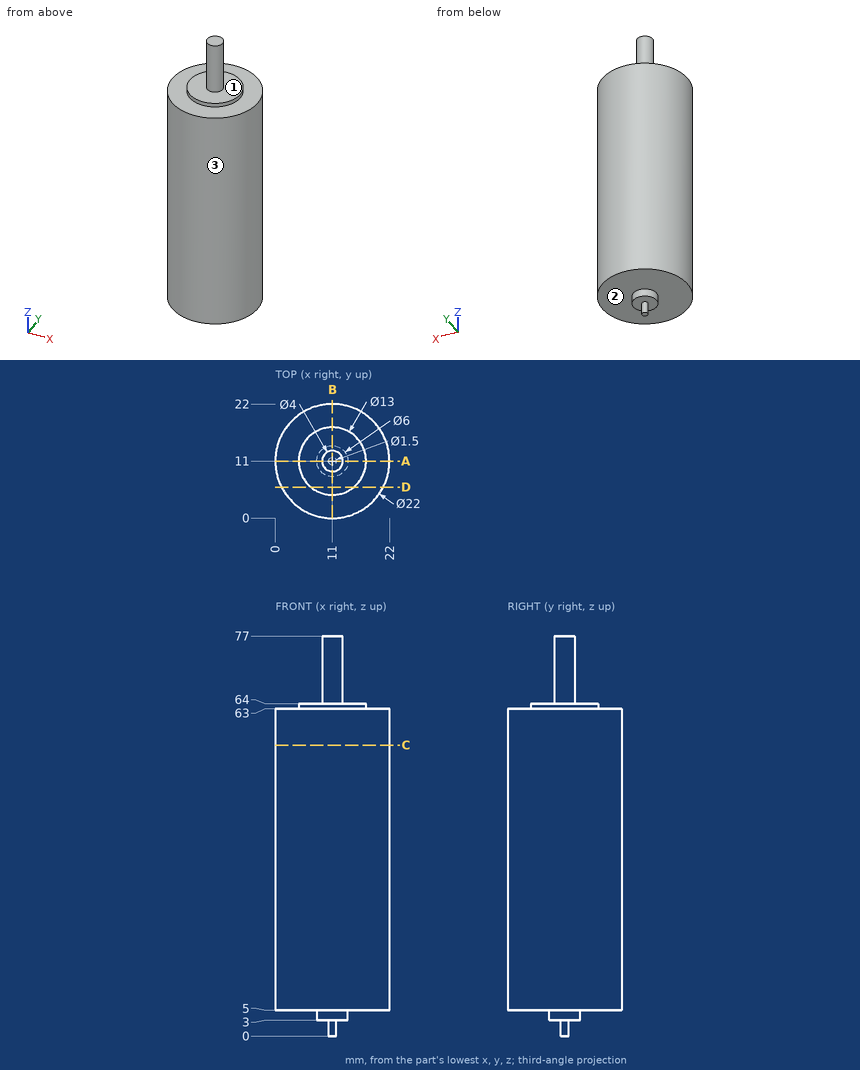
Print and shaded views of the part. All mm, measured from the part's lowest x, y and z. A direction names the side the tool comes from. Give positions to 0.01 mm unless a question says otherwise; leave off trailing zeros. Loops run counter-clockwise (first coordinate to the right, second up) from the corner with the lowest first, then second, coordinate; pieces in that order, holes last. Notation, with made-up numbers: (54.25, 32) -> (98.25, 32) arc R19 ccw to (98.25, 60) -> close; hole circle Ø7 at (-29, 38). An arc over 180 degrees is marked (long way). Use CSV: the item, a comma, the result in double quotes. Start each with the question number.
1) Tool access for the marked faces 1, 2 and 3: list every direction of +Z, -Z, +X, -X, +Y, -Y with a clear straight run to the whole face (end or side of a thin tool).
2) Wall check: line 1 (Z direction, x = 9.5, y = 2.75); line 2 (Z direction, x = 10, y = 9); line 3 (Y direction, x = 11.5, z = 13). Give the ranges that are in metal, low to high.
3) Flat gauge pins, fed straight in: pin 1 Ø8 at (x, y) = (17.5, 13.5) entering from +Z; pin 2 Ø4 at (x, y) = (10, 17) entering from -Z; pin 3 Ø2 at (x, z) = (19.5, 10) entering from +Y. Where does each tip first touch, or does it go through?
4) Slice it at A-A on y = 11. Give the cut face in (x, z), plus the area to 3 significant figures.
5) Slice it at D-D on y = 6. Give the cut face in (x, z).
6) Slice it at C-C on z = 56. Give the cut face in (x, y).
Computed values:
1,face 1,"+Z"
1,face 2,"-Z"
1,face 3,"+Z, -Z"
2,line 1,"z = 5 to 63"
2,line 2,"z = 3 to 64"
2,line 3,"y = 0.01 to 21.99"
3,pin 1,"stops at z = 64"
3,pin 2,"stops at z = 5"
3,pin 3,"stops at y = 19.05"
4,outline,"(0, 5) -> (8, 5) -> (8, 3) -> (10.25, 3) -> (10.25, 0) -> (11.75, 0) -> (11.75, 3) -> (14, 3) -> (14, 5) -> (22, 5) -> (22, 63) -> (17.5, 63) -> (17.5, 64) -> (13, 64) -> (13, 77) -> (9, 77) -> (9, 64) -> (4.5, 64) -> (4.5, 63) -> (0, 63) -> close"
4,area,"1,360 mm^2"
5,outline,"(1.2, 5) -> (20.8, 5) -> (20.8, 63) -> (15.15, 63) -> (15.15, 64) -> (6.85, 64) -> (6.85, 63) -> (1.2, 63) -> close"
6,outline,"circle Ø22 at (11, 11)"
